For this review, take the finished solid that the model builds, in its own axes (mm). Face numbers are marked on the shaded views. A direction names the side the tool comes from. Round coordinates to 2 decimals unless told otherwise and drop trailing zeros. Write each loop counter-clockwise with the first axis right and the second up, starting at its lowest first coordinate (ties: lowest second). Pieces come first, ordered by that corner, then holes.
from build123d import *

# Parameters (mm, degrees)
RESSALTO_EXTRUS_O1_DEPTH = 80
RESSALTO_EXTRUS_O2_DEPTH = 80
ESBO_O3_R                = 15
ESBO_O3_R_2              = 20
CORTE_EXTRUS_O2_DEPTH    = 131


with BuildPart() as part:
    # Esboço1 → Ressalto-extrusão1 (new body, symmetric)
    with BuildSketch(Plane.XY):
        Polygon((-110.350506682, 0), (39.649493318, 0), (39.649493318, 80), (179.649493318, 80), (179.649493318, 30), (89.649493318, 30), (89.649493318, -50), (-110.350506682, -50), align=None)
    extrude(amount=RESSALTO_EXTRUS_O1_DEPTH, both=True)

    # Esboço2 → Ressalto-extrusão2 (add)
    with BuildSketch(Plane(origin=(0, 0, 0), x_dir=(1, 0, 0), z_dir=(0, 1, 0))):
        with BuildLine():
            Line((9.649493318, 45), (39.649493318, 45))
            Line((39.649493318, 45), (39.649493318, -45))
            Line((39.649493318, -45), (9.649493318, -45))
            ThreePointArc((9.649493318, -45), (-35.350506682, 0), (9.649493318, 45))
        make_face()
    extrude(amount=RESSALTO_EXTRUS_O2_DEPTH)

    # Esboço3 → Corte-extrusão2 (cut, through all)
    with BuildSketch(Plane(origin=(0, 80, 0), x_dir=(1, 0, 0), z_dir=(0, 1, 0))):
        with Locations((-70.350506682, 40)):
            Circle(ESBO_O3_R)
        with Locations((139.649493318, 40)):
            Circle(ESBO_O3_R)
        with Locations((139.649493318, -40)):
            Circle(ESBO_O3_R)
        with Locations((-70.350506682, -40)):
            Circle(ESBO_O3_R)
        with Locations((9.649493318, 0)):
            Circle(ESBO_O3_R_2)
    extrude(amount=-CORTE_EXTRUS_O2_DEPTH, mode=Mode.SUBTRACT)


solid = part.part
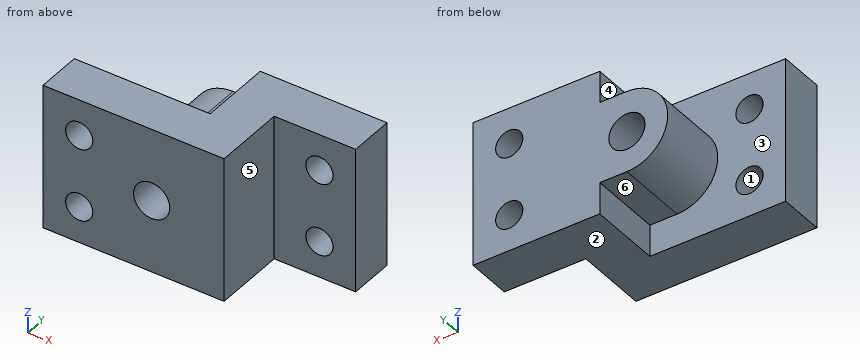
(1) For line 1 along X through (y, z) = (-25.5, -40); line 2 along Y through (x, z) = (159, 63.5); line 3 along X through (y, z) = (-14.5, -39), list the stretches that pass through material, from the lowest coordinate up.
Geometry check:
line 1: x = -110.35 to -85.35, -55.35 to 89.65
line 2: y = 30 to 80
line 3: x = -110.35 to -85.32, -55.38 to 89.65
(2) For the marked faces 4, 5 and 6, list the 3-axis set-ups (+Z, -Z, +X, -X, +Y, -Y) from which the entire face can be reached by the end or side of a thin tool; tool diameter is ignored.
Geometry check:
face 4: +Z, -X, +Y
face 5: +Z, -Z, +X, -Y
face 6: -Z, -X, +Y
(3) For pin 1 Ø24 at (y, z) = (5.5, -20) entering from +X; pin 2 Ø10.5 at (y, z) = (45.5, -63) entering from -X, all flat-tipped, find the tip position at first contact; note any pin that passes through.
Geometry check:
pin 1: stops at x = 89.65
pin 2: stops at x = 39.65
(4) Mouldability with a two-part tool opening along Z and no side actions: class the marked faces 1, 2 and 3 as pulls with the +Z half, pulls with the -Z half, needs draft (parallel to the pull), parting line crosses it, or undercut.
Geometry check:
face 1: undercut
face 2: pulls with the -Z half
face 3: needs draft
(5) We need section D-D, the plane z = -40. Give the boundary of the cut face in (x, y), and give its area (3 significant figures).
Geometry check:
outline: (-110.35, -50) - (-85.35, -50) - (-85.35, 0) - (-110.35, 0) - close; (-55.35, -50) - (89.65, -50) - (89.65, 30) - (124.65, 30) - (124.65, 80) - (-10.97, 80) - (-10.97, 0) - (-55.35, 0) - close; (154.65, 30) - (179.65, 30) - (179.65, 80) - (154.65, 80) - close
area: 19,500 mm2
(6) We need section C-C, the plane x = 147. Give the boundary of the cut face in (y, z).
Geometry check:
outline: (30, -80) - (80, -80) - (80, -53.08) - (30, -53.08) - close; (30, -26.92) - (80, -26.92) - (80, 26.92) - (30, 26.92) - close; (30, 53.08) - (80, 53.08) - (80, 80) - (30, 80) - close
(7) We need section A-A, the plane z = 0. Give the boundary of the cut face in (x, y), and give its area (3 significant figures).
Geometry check:
outline: (-110.35, -50) - (-10.35, -50) - (-10.35, 80) - (-35.35, 80) - (-35.35, 0) - (-110.35, 0) - close; (29.65, -50) - (89.65, -50) - (89.65, 30) - (179.65, 30) - (179.65, 80) - (29.65, 80) - close
area: 19,300 mm2
(8) We need section B-B, the plane y = 54. Give the boundary of the cut face in (x, z), and give its area (3 significant figures).
Geometry check:
outline: (9.65, -45) - (39.65, -45) - (39.65, -80) - (179.65, -80) - (179.65, 80) - (39.65, 80) - (39.65, 45) - (9.65, 45) arc R45 ccw to start; hole circle Ø40 at (9.65, 0); hole circle Ø30 at (139.65, -40); hole circle Ø30 at (139.65, 40)
area: 25,600 mm2
